Here's the drawing with two shaded views (mm, measured from the low corner). I have some questions. Coordinates: 2 decimals unless noted, no trailing zeros. Loops run counter-clockwise (first coordinate to the right, second up) from the corner with the lowest first, then second, coordinate; pieces in that order, holes last.
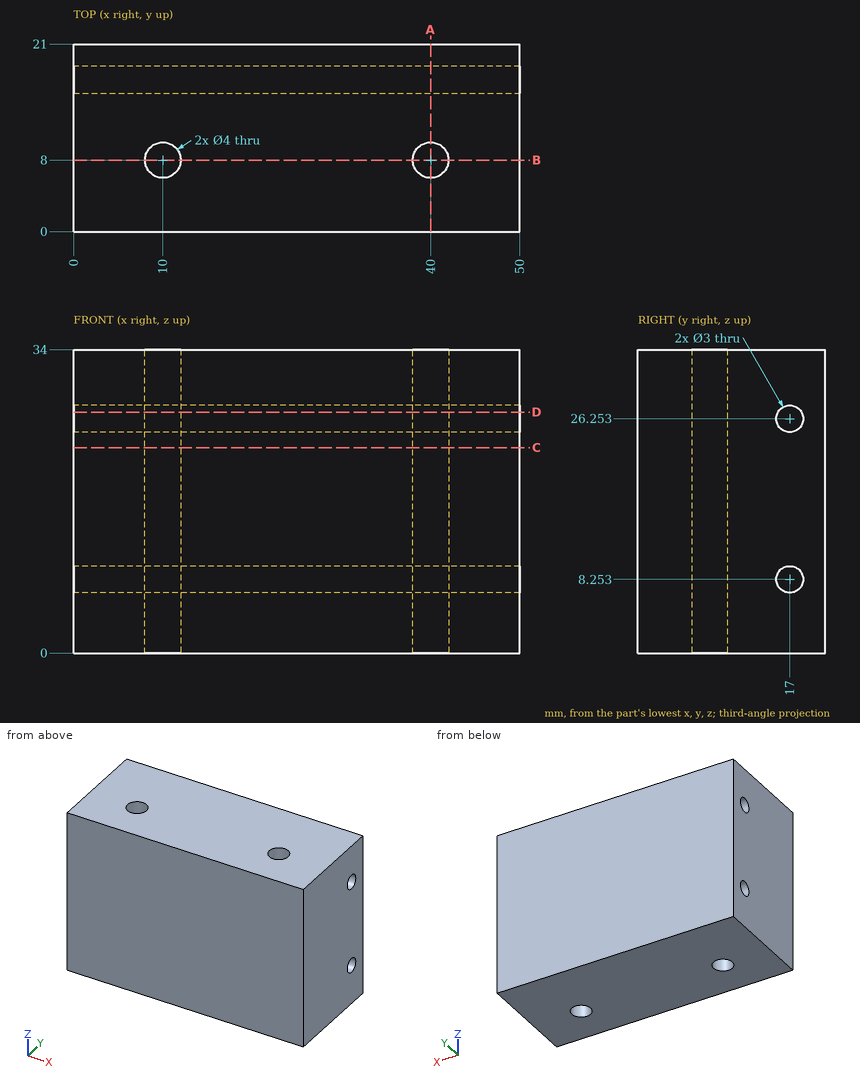
(1) I'm going to push a flat-ended pin straight in: pin 1 (3.5 mm diameter, centred on y = 17, z = 8.25, fed in from -X). Where does the tip first touch, or does it pass through?
Check values:
pin 1: stops at x = 0
(2) I want a section at D-D on z = 27. Write out the boundary of the cut face in (x, y), then the cut area to 3 significant figures.
Check values:
outline: (0, 0) - (50, 0) - (50, 15.7) - (0, 15.7) - close; (0, 18.3) - (50, 18.3) - (50, 21) - (0, 21) - close; hole circle Ø4 at (10, 8); hole circle Ø4 at (40, 8)
area: 895 mm2
(3) I want a section at B-B on y = 8. Write out the boundary of the cut face in (x, z).
Check values:
outline: (0, 0) - (8, 0) - (8, 34) - (0, 34) - close; (12, 0) - (38, 0) - (38, 34) - (12, 34) - close; (42, 0) - (50, 0) - (50, 34) - (42, 34) - close
(4) If I drill on probe 1 along Z at (x, y) = (19, 17); probe 2 along X at (y, z) = (7.5, 8); probe 3 along Y at (x, z) = (40, 9.5) (1 decimal), over which ranges is the centre line in solid material (lowest first)?
Check values:
probe 1: z = 0 to 6.75, 9.75 to 24.75, 27.75 to 34
probe 2: x = 0 to 8.06, 11.94 to 38.06, 41.94 to 50
probe 3: y = 0 to 6, 10 to 16.2, 17.8 to 21
(5) I want a section at A-A on x = 40. Write out the boundary of the cut face in (y, z), then the cut area to 3 significant figures.
Check values:
outline: (0, 0) - (6, 0) - (6, 34) - (0, 34) - close; (10, 0) - (21, 0) - (21, 34) - (10, 34) - close; hole circle Ø3 at (17, 8.25); hole circle Ø3 at (17, 26.25)
area: 564 mm2
(6) I want a section at C-C on z = 23. Write out the boundary of the cut face in (x, y).
Check values:
outline: (0, 0) - (50, 0) - (50, 21) - (0, 21) - close; hole circle Ø4 at (10, 8); hole circle Ø4 at (40, 8)
